from build123d import *

# Parameters (mm, degrees)
SKETCH1_R           = 75
SKETCH1_R_2         = 10
BOSS_EXTRUDE1_DEPTH = 30
SKETCH2_R           = 20
BOSS_EXTRUDE2_DEPTH = 30
BOSS_EXTRUDE5_DEPTH = 60
CUT_EXTRUDE1_DEPTH  = 23


with BuildPart() as part:
    # Sketch1 → Boss-Extrude1 (new body)
    with BuildSketch(Plane(origin=(0, 0, 0), x_dir=(1, 0, 0), z_dir=(0, 1, 0))):
        Circle(SKETCH1_R)
        with Locations((0, -51.940298755)):
            Circle(SKETCH1_R_2, mode=Mode.SUBTRACT)
        with Locations((52.648575556, 0)):
            Circle(SKETCH1_R_2, mode=Mode.SUBTRACT)
        with Locations((-52.648575556, 0)):
            Circle(SKETCH1_R_2, mode=Mode.SUBTRACT)
        with Locations((0, 51.940298755)):
            Circle(SKETCH1_R_2, mode=Mode.SUBTRACT)
    extrude(amount=-BOSS_EXTRUDE1_DEPTH)

    # Sketch2 → Boss-Extrude2 (add)
    with BuildSketch(Plane.XZ.offset(30)):
        Circle(SKETCH2_R)
    extrude(amount=BOSS_EXTRUDE2_DEPTH)

    # Sketch3 → Boss-Extrude5 (add, through all)
    with BuildSketch(Plane.XZ.offset(60)):
        Polygon((2.130897014, 4.097878872), (-2.483418698, 3.894350383), (-4.614315712, -0.20352849), (-2.130897014, -4.097878872), (2.483418698, -3.894350383), (4.614315712, 0.20352849), align=None)
    extrude(amount=-BOSS_EXTRUDE5_DEPTH)

    # Sketch3<3> → Cut-Extrude1 (cut)
    with BuildSketch(Plane.XZ.offset(60)):
        Polygon((2.130897014, 4.097878872), (-2.483418698, 3.894350383), (-4.614315712, -0.20352849), (-2.130897014, -4.097878872), (2.483418698, -3.894350383), (4.614315712, 0.20352849), align=None)
    extrude(amount=-CUT_EXTRUDE1_DEPTH, mode=Mode.SUBTRACT)


solid = part.part
Input: part model. Units: mm. Frame: model coordinates. A direction names the side the tool comes from. Coordinates: 2 decimals unless noted, no trailing zeros. Loops run counter-clockwise (first coordinate to the right, second up) from the corner with the lowest first, then second, coordinate; pieces in that order, holes last.
(1) Section D-D on y = -16. Return the cut outline in (x, z), then the cut area to 3 significant figures.
(2) Pull-direction query (X, two-part tool) for faces 3 (the face through (3.534, -48.661, -1.874)), 4 (the face through (-9.764, -14.79, -74.362)), 5 (the face through (16, -30, 16)), 6 (the face through (-1.302, -14.79, -61.855)); classes: released by +X, released by -X, zero draft, split by the parting line, or undercut.
(3) First-contact query: pin 1 Ø16 at (x, z) = (0, -51.94) entering from -Y; pin 2 Ø23 at (x, z) = (-52.65, 0) entering from -Y; pin 3 Ø8 at (y, z) = (-18.5, 12.5) entering from +X; pin 4 Ø12 at (x, y) = (-51.5, -33) entering from -Z. Flat tips, straight axial feed; report the tip coordinate or a pass-through.
(4) Set-up query: faces 1 (the face through (-0.3, -60, -4.2)), 2 (the face through (-4.336, -44.79, -19.524)). Return all of +Z, -Z, +X, -X, +Y, -Y with unobstructed straight access to the full face (end or side cutting, diameter ignored); none if empty.
(5) Section A-A on y = -46. Return the cut outline in (x, z), then the cut area to 3 significant figures.
(6) Material intervals for probe 1 along Z at (x, y) = (0, -19.25); probe 2 along X at (y, z) = (-21, 0); probe 3 along Z at (x, y) = (5.5, -19.5), sorted ascending.
(7) Section B-B on x = 0. Return the cut outline in (y, z).
(8) Section C-C on x = 57.5. Return the cut outline in (y, z), then the cut area to 3 significant figures.
Data:
1. outline: circle Ø150 at (0, 0); hole circle Ø20 at (-52.65, 0); hole circle Ø20 at (0, -51.94); hole circle Ø20 at (0, 51.94); hole circle Ø20 at (52.65, 0)
1. area: 16,400 mm2
2. face 3: undercut
2. face 4: split by the parting line
2. face 5: zero draft
2. face 6: undercut
3. pin 1: passes through
3. pin 2: stops at y = -30
3. pin 3: stops at x = 74.52
3. pin 4: stops at z = -59
4. face 1: +Z, -Z, +X, -X, -Y
4. face 2: -Y
5. outline: circle Ø40 at (0, 0); hole (-4.61, -0.2) - (-2.13, -4.1) - (2.48, -3.89) - (4.61, 0.2) - (2.13, 4.1) - (-2.48, 3.89) - close
5. area: 1,200 mm2
6. probe 1: z = -75 to -61.94, -41.94 to 41.94, 61.94 to 75
6. probe 2: x = -75 to -62.65, -42.65 to 42.65, 62.65 to 75
6. probe 3: z = -74.8 to -60.29, -43.59 to 43.59, 60.29 to 74.8
7. outline: (-60, -20) - (-30, -20) - (-30, -41.94) - (0, -41.94) - (0, 41.94) - (-30, 41.94) - (-30, 20) - (-60, 20) - (-60, 4) - (-37, 4) - (-37, -4) - (-60, -4) - close; (-30, -75) - (0, -75) - (0, -61.94) - (-30, -61.94) - close; (-30, 61.94) - (0, 61.94) - (0, 75) - (-30, 75) - close
8. outline: (-30, -48.15) - (0, -48.15) - (0, -8.74) - (-30, -8.74) - close; (-30, 8.74) - (0, 8.74) - (0, 48.15) - (-30, 48.15) - close
8. area: 2,360 mm2
